Work out the finished part from the listing and answer in its coordinate system (mm). Round coordinates to 2 decimals unless told otherwise and drop trailing zeros. Order: outer loops, then holes, each group sorted by start corner. A loop starts at its lowest first (then second) coordinate and runs counter-clockwise, first axis right, second up.
Autodesk Inventor part; units mm, degrees
ref_plane "to_cap_XY" through (0, 38, 0) normal (0, -1, 0) x (1, 0, 0)
ref_plane "to_cap_YZ" through (0, 38, 0) normal (1, 0, 0) x (0, 0, 1)
ref_plane "to_cap_ZX" through (0, 38, 0) normal (0, 0, 1) x (0, -1, 0)
sketch "Sketch_1" plane through (0, 0, 0) normal (0, 0, 1) x (1, 0, 0)
  line L0 (0, -38) -> (0, 38)
  line L1 (0, 32) -> (3, 32)
  line L2 (3, 32) -> (4, 31)
  line L3 (4, 31) -> (4, 1)
  line L4 (4, 1) -> (3, 0)
  line L5 (3, 0) -> (3, -5.8)
  line L6 (3, -5.8) -> (2.8, -6)
  line L7 (2.8, -6) -> (0, -6)
  line L8 (0, -6) -> (0, 32)
revolve "Revolution1" add sketch "Sketch_1" angle 360 about axis through (0, -38, 0) along (0, -1, 0)
thread "Thread1"
sketch "Sketch2" plane through (0, 32, 0) normal (0, 1, 0) x (1, 0, 0)
  point P0 (0, 0)
hole "Hole1" at (0, 32, 0) direction (0, -1, 0) diameter 2.9 depth 20 tip angle 118
ref_plane "to_cap_XY" through (0, 38, 0) normal (0, -1, 0) x (1, 0, 0)
ref_plane "to_cap_YZ" through (0, 38, 0) normal (1, 0, 0) x (0, 0, 1)
ref_plane "to_cap_ZX" through (0, 38, 0) normal (0, 0, 1) x (0, -1, 0)
ref_plane "to_nut1_XY" through (0, 7, 0) normal (0, -1, 0) x (1, 0, 0)
ref_plane "to_nut1_YZ" through (0, 7, 0) normal (1, 0, 0) x (0, 0, 1)
ref_plane "to_nut1_ZX" through (0, 7, 0) normal (0, 0, 1) x (0, -1, 0)
ref_plane "to_nut2_XY" through (0, 23, 0) normal (0, -1, 0) x (1, 0, 0)
ref_plane "to_nut2_YZ" through (0, 23, 0) normal (1, 0, 0) x (0, 0, 1)
ref_plane "to_nut2_ZX" through (0, 23, 0) normal (0, 0, 1) x (0, -1, 0)
ref_plane "to_rod_XY" through (0, 32, 0) normal (0, 1, 0) x (1, 0, 0)
ref_plane "to_rod_YZ" through (0, 32, 0) normal (1, 0, 0) x (0, 0, -1)
ref_plane "to_rod_ZX" through (0, 32, 0) normal (0, 0, -1) x (0, 1, 0)
ref_plane "to_washers_1_XY" through (0, 15, 0) normal (0, 1, 0) x (1, 0, 0)
ref_plane "to_washers_1_YZ" through (0, 15, 0) normal (1, 0, 0) x (0, 0, -1)
ref_plane "to_washers_1_ZX" through (0, 15, 0) normal (0, 0, -1) x (0, 1, 0)
ref_plane "to_washers_2_XY" through (0, 17, 0) normal (0, -1, 0) x (1, 0, 0)
ref_plane "to_washers_2_YZ" through (0, 17, 0) normal (1, 0, 0) x (0, 0, 1)
ref_plane "to_washers_2_ZX" through (0, 17, 0) normal (0, 0, 1) x (0, -1, 0)
properties part number "C-AC0806M_b"
Item 1: Find the intervals of material crossed by line 1 along Z through (x, y) = (0, 17.75); line 2 along X through (y, z) = (22.5, 1); line 3 along X through (y, z) = (5.5, -1.5), in increasing order.
Item 2: For a pull along Z with two mould halves and no side action, classify faces 1 (the face through (-3, -3, 0)), 2 (the face through (-0.06, 21.86, -1.45)), 3 (the face through (0, -6, 0)) as released by +Z, released by -Z, zero draft, split by the parting line, or undercut.
Item 3: Find section A-A (y = 20). Write down the section's boundary in (x, z), plus the area to 3 significant figures.
Item 4: Given pin 1 (1 mm diameter, centred on x = 1.5, y = 8.5, fed in from -Z); pin 2 (3 mm diameter, centred on y = 11.5, z = 3, fed in from +X); pin 3 (2.5 mm diameter, centred on x = 0, z = 0, fed in from +Y), each flat-ended and moving along its own axis, determine where each tip first touches the part or whether it passes through.
Model answer:
1. line 1: z = -4 to -1.45, 1.45 to 4
1. line 2: x = -3.87 to -1.05, 1.05 to 3.87
1. line 3: x = -3.71 to 3.71
2. face 1: split by the parting line
2. face 2: undercut
2. face 3: zero draft
3. outline: circle Ø8 at (0, 0); hole circle Ø2.9 at (0, 0)
3. area: 43.7 mm2
4. pin 1: stops at z = -3.87
4. pin 2: stops at x = 3.71
4. pin 3: stops at y = 11.88
